Geometry: final body of the model. Coordinates: model frame, mm. Give positions to 0.01 mm unless a question says otherwise; leave off trailing zeros. Order: outer loops, then holes, each group sorted by start corner. A loop starts at its lowest first (then second) coordinate and runs counter-clockwise, first axis right, second up. Notation, with made-up numbers: M 56.5,64.5 L 80.5,64.5 A5 ccw 80.5,71.5 Z; hole C 26,-9 d7. An arc over 180 degrees is marked long. Write item = value, one per line. Start each with the question number.
from build123d import *

# Parameters (mm, degrees)
ESQUISSE1_W             = 0.6
ESQUISSE1_H             = 0.6
BOSS_EXTRU_1_DEPTH      = 2.8
ESQUISSE2_W             = 0.6
ESQUISSE2_H             = 0.575
ENL_V_MAT_EXTRU_1_DEPTH = 1
BOSS_EXTRU_2_DEPTH      = 4
BOSS_EXTRU_2_DEPTH_BACK = 7.8
ESQUISSE3_W             = 0.6
ESQUISSE3_H             = 0.6
CHANFREIN1_SIZE         = 0.2
ESQUISSE4_R             = 0.674645205
ESQUISSE4_R_2           = 0.5
BOSS_EXTRU_3_DEPTH      = 0.01


with BuildPart() as part:
    # Esquisse1 → Boss.-Extru.1 (new body)
    with BuildSketch(Plane.XY):
        Polygon((-0.675, 0.875), (-0.875, 0.675), (-0.875, -0.675), (-0.675, -0.875), (0.675, -0.875), (0.875, -0.675), (0.875, 0.675), (0.675, 0.875), align=None)
        Rectangle(ESQUISSE1_W, ESQUISSE1_H, mode=Mode.SUBTRACT)
    extrude(amount=BOSS_EXTRU_1_DEPTH)

    # Esquisse2 → Enlèv. mat.-Extru.1 (cut)
    with BuildSketch(Plane.XY.offset(2.8)):
        with Locations((0, -0.5875)):
            Rectangle(ESQUISSE2_W, ESQUISSE2_H)
    extrude(amount=-ENL_V_MAT_EXTRU_1_DEPTH, mode=Mode.SUBTRACT)

    # Esquisse3 → Boss.-Extru.2 (add, two sides: drawn at the far end of the back side and taken through both)
    with BuildSketch(Plane.XY.offset(2.8).offset(-BOSS_EXTRU_2_DEPTH_BACK)):
        Rectangle(ESQUISSE3_W, ESQUISSE3_H)
    extrude(amount=BOSS_EXTRU_2_DEPTH + BOSS_EXTRU_2_DEPTH_BACK)

    # Chanfrein1
    chanfrein1_edges = [part.edges().sort_by_distance(p)[0] for p in [
        (0, -0.3, -5),
        (0.3, 0, -5),
        (-0.3, 0, -5),
        (0, 0.3, -5),
        (0.3, 0, 6.8),
        (0, 0.3, 6.8),
        (-0.3, 0, 6.8),
        (0, -0.3, 6.8),
    ]]
    chamfer(chanfrein1_edges, length=CHANFREIN1_SIZE)

    # Esquisse4 → Boss.-Extru.3 (add)
    with BuildSketch(Plane.XY.offset(2.8)):
        with Locations(Location((0, 0, 0), (0, 0, 243.597249523))):
            Circle(ESQUISSE4_R)
        with Locations(Location((0, 0, 0), (0, 0, 233.130102354))):
            Circle(ESQUISSE4_R_2, mode=Mode.SUBTRACT)
    extrude(amount=BOSS_EXTRU_3_DEPTH)


solid = part.part
1) Cut plane C-C (y = 0). Return loops of the section in (x, z) (3 decimals).
2) Cut plane B-B (z = 2). Return loops of the section in (x, y) (3 decimals).
3) Cut plane A-A (x = 0). Return loops of the section in (y, z) (3 decimals).
4) Pin query (flat end, axial travel): pin 1 Ø0.7 at (y, z) = (0, -2.5) entering from -X; pin 2 Ø0.5 at (x, y) = (0, -0.5) entering from +Z; pin 3 Ø0.5 at (x, y) = (0, -0.5) entering from -Z. Return the tip coordinate at first contact, or that it passes through.
5) Ray query, L1, parallel to Y at x = -0.2, z = -1.75; L2, parallel to Y at x = -0.1, z = 2.25 (3 decimals); L3, parallel to Z at x = 0.7, y = -0.6. Return the intervals inside material, ascending.
Reply:
q1.outline = M -0.875,0 L -0.3,0 L -0.3,-4.8 L -0.1,-5 L 0.1,-5 L 0.3,-4.8 L 0.3,0 L 0.875,0 L 0.875,2.8 L 0.675,2.8 L 0.675,2.81 L 0.5,2.81 L 0.5,2.8 L 0.3,2.8 L 0.3,6.6 L 0.1,6.8 L -0.1,6.8 L -0.3,6.6 L -0.3,2.8 L -0.5,2.8 L -0.5,2.81 L -0.675,2.81 L -0.675,2.8 L -0.875,2.8 Z
q2.outline = M -0.875,-0.675 L -0.675,-0.875 L -0.3,-0.875 L -0.3,-0.3 L 0.3,-0.3 L 0.3,-0.875 L 0.675,-0.875 L 0.875,-0.675 L 0.875,0.675 L 0.675,0.875 L -0.675,0.875 L -0.875,0.675 Z
q3.outline = M -0.875,0 L -0.3,0 L -0.3,-4.8 L -0.1,-5 L 0.1,-5 L 0.3,-4.8 L 0.3,0 L 0.875,0 L 0.875,2.8 L 0.675,2.8 L 0.675,2.81 L 0.5,2.81 L 0.5,2.8 L 0.3,2.8 L 0.3,6.6 L 0.1,6.8 L -0.1,6.8 L -0.3,6.6 L -0.3,1.8 L -0.875,1.8 Z; M -0.675,2.8 L -0.5,2.8 L -0.5,2.81 L -0.675,2.81 Z
q4.pin_1 = -0.3
q4.pin_2 = 6.65
q4.pin_3 = -4.85
q5.L1 = -0.3 to 0.3
q5.L2 = -0.3 to 0.875
q5.L3 = 0 to 2.8
